from build123d import *

# Parameters (mm, degrees)
SKETCH_1_R               = 4
EXTRUDE_1_DEPTH          = 30
SKETCH_2_R               = 2
CUT_EXTRUDE_1_DEPTH      = 8
CUT_EXTRUDE_2_DEPTH      = 41.902322672
CUT_EXTRUDE_2_DEPTH_BACK = 41.902322672
SKETCH_4_R               = 1.7


with BuildPart() as part:
    # 草图1 → 凸台-拉伸1 (new body)
    with BuildSketch(Plane.XY):
        Polygon((17, 11), (-17, 11), (-17, 5), (-16.130865539, 3.691288487), (-16.130865539, -7), (-7.678245569, -7), (-5.021787053, -11), (5.021787053, -11), (7.678245569, -7), (16.130865539, -7), (16.130865539, 3.691288487), (17, 5), align=None)
        Circle(SKETCH_1_R, mode=Mode.SUBTRACT)
    extrude(amount=EXTRUDE_1_DEPTH)

    # 草图2 → 切除-拉伸1 (cut)
    with BuildSketch(Plane(origin=(0, 11, 0), x_dir=(1, 0, 0), z_dir=(0, 1, 0))):
        with Locations(Location((-12, -6, 0), (0, 0, 270))):
            Circle(SKETCH_2_R)
        with Locations(Location((-12, -24, 0), (0, 0, 270))):
            Circle(SKETCH_2_R)
        with Locations(Location((12, -6, 0), (0, 0, 270))):
            Circle(SKETCH_2_R)
        with Locations(Location((12, -24, 0), (0, 0, 270))):
            Circle(SKETCH_2_R)
    extrude(amount=-CUT_EXTRUDE_1_DEPTH, mode=Mode.SUBTRACT)

    # 草图4 → 切除-拉伸2 (cut, two sides: drawn at the far end of the back side and taken through both)
    with BuildSketch(Plane(origin=(0, 11, 0), x_dir=(1, 0, 0), z_dir=(0, 1, 0)).offset(-CUT_EXTRUDE_2_DEPTH_BACK)):
        with Locations(Location((-12, -6, 0), (0, 0, 270))):
            Circle(SKETCH_4_R)
        with Locations(Location((-12, -24, 0), (0, 0, 270))):
            Circle(SKETCH_4_R)
        with Locations(Location((12, -6, 0), (0, 0, 270))):
            Circle(SKETCH_4_R)
        with Locations(Location((12, -24, 0), (0, 0, 270))):
            Circle(SKETCH_4_R)
    extrude(amount=CUT_EXTRUDE_2_DEPTH + CUT_EXTRUDE_2_DEPTH_BACK, mode=Mode.SUBTRACT)


solid = part.part
Input: part model. Units: mm. Frame: model coordinates. A direction names the side the tool comes from. Give positions to 0.01 mm unless a question says otherwise; leave off trailing zeros. Write each loop counter-clockwise with the first axis right and the second up, starting at its lowest first coordinate (ties: lowest second). Pieces come first, ordered by that corner, then holes. Notation, with made-up numbers: M 73.25,81.25 L 109.25,81.25 A24 ccw 109.25,108.25 Z; hole C 11,83.5 d9. An arc over 180 degrees is marked long. Write item = value, one per line. Start each with the question number.
1) Cut plane A-A on z = 24. Count the separate pieces of the cut face and the enclosed holes in it, then the cut area to 3 significant figures.
2) Material intervals for line 1 along Z through (x, y) = (12, -1.5); line 2 along X through (y, z) = (6.5, 24); line 3 along X through (y, z) = (-6, 25.5), sorted ascending. Write a range as [from, to].
3) Cut plane C-C on x = 12. Return the cut outline in (y, z).
4) Cut plane B-B on y = 0. Return the cut outline in (x, z).
5) Reachability of faces 1 (the cylindrical face through (14, 7, 6)), 2 (the flat face through (6.33, -9.03, 14.79)) from +Z, -Z, +X, -X, +Y, -Y: full face, straight path, thin tool, end or side. Return the list, or none.
6) First-contact query: pin 1 Ø7 at (x, y) = (0, 0) entering from -Z; pin 2 Ø4 at (x, z) = (-12, 6) entering from -Y; pin 3 Ø3 at (x, z) = (-13, 24) entering from +Y; pin 4 Ø2 at (y, z) = (-7.5, 25) entering from +X. Flat tips, straight axial feed; report the tip coordinate or a pass-through.
7) Draft query along Z for faces 3 (the cylindrical face through (-13.66, -2.07, 5.63)), 4 (the flat face through (-6.37, -8.97, 14.79)), 5 (the flat face through (0, 5, 0)). Return one class per face: +Z half, -Z half, draft (parallel to the pull), parting line (faces both ways), or undercut.
8) Cut plane D-D on y = 7.5. Return the cut outline in (x, z), then the cut area to 3 significant figures.
Solved:
q1.separate_pieces = 3
q1.enclosed_holes = 1
q1.area = 461 mm2
q2.line_1 = [0, 4.3], [7.7, 22.3], [25.7, 30]
q2.line_2 = [-17, -14], [-10, 10], [14, 17]
q2.line_3 = [-16.13, -12.8], [-11.2, 11.2], [12.8, 16.13]
q3.outline = M -7,0 L 11,0 L 11,4 L 3,4 L 3,4.3 L -7,4.3 Z; M -7,7.7 L 3,7.7 L 3,8 L 11,8 L 11,22 L 3,22 L 3,22.3 L -7,22.3 Z; M -7,25.7 L 3,25.7 L 3,26 L 11,26 L 11,30 L -7,30 Z
q4.outline = M -16.13,0 L -4,0 L -4,30 L -16.13,30 Z; M 4,0 L 16.13,0 L 16.13,30 L 4,30 Z; hole C -12,6 d3.4; hole C -12,24 d3.4; hole C 12,6 d3.4; hole C 12,24 d3.4
q5.face_1 = +Y
q5.face_2 = +Z, -Z, +X, -Y
q6.pin_1 = through
q6.pin_2 = -7
q6.pin_3 = 11
q6.pin_4 = 16.13
q7.face_3 = undercut
q7.face_4 = draft
q7.face_5 = -Z half
q8.outline = M -17,0 L 17,0 L 17,30 L -17,30 Z; hole C -12,6 d4; hole C -12,24 d4; hole C 12,6 d4; hole C 12,24 d4
q8.area = 970 mm2
